Check sheet for the modelled part. Datum: model origin and axes. Units: mm. A direction names the side the tool comes from. Give positions to 0.01 mm unless a question says otherwise; leave off trailing zeros. Write each loop counter-clockwise with the first axis right and the second up, starting at its lowest first coordinate (ties: lowest second). Pieces come first, ordered by that corner, then holes. Notation, with made-up numbers: M 19.5,59 L 31.5,59 A16 ccw 31.5,66 Z; hole C 5,-13 d8. An arc over 180 degrees is marked long. Use CSV: the item, a comma, the result in double quotes. Start each with the question number.
1. Scan lines: line 1 (X direction, y = 7.25, z = 87.5); line 2 (Z direction, x = -2.5, y = 5.5); line 3 (X direction, y = 3.75, z = 87.5). Record each from-to range of solid material in increasing order.
2. Mould release check, pull along Z, two halves, no side actions. Record for faces 1 (the face through (23, 5.2, 49)), 2 (the face through (6, 5, 100)), 3 (the face through (-2.41, 4.93, 85.14)): +Z half, -Z half, draft (parallel to the pull), parting line (faces both ways), or undercut.
3. Cross-section at C-C, the plane z = 76. Enter the section's corners in (x, y).
4. Access from +Z, -Z, +X, -X, +Y, -Y to the whole of each face (thin tool, end or side, straight path). Record for faces 4 (the face through (17.32, 2.56, 98.5)), 5 (the face through (18.75, 3, 49)), 6 (the face through (17.25, 2.56, 1.43)).
5. Cross-section at B-B, the plane y = 7.5. Enter the section's corners in (x, z).
6. Cross-section at D-D, the plane z = 13. Enter the section's corners in (x, y), and give its area (3 significant figures).
7. Cross-section at A-A, the plane z = 87.5. Enter the section's corners in (x, y).
8. Depth check by flat-ended pin: P1, Ø12.5, axis at x = 18, z = 51.5, coming from the -Y side; P2, Ø5, axis at x = -0.25, z = 87.5, coming from the -Y side; P3, Ø3, axis at y = 1, z = 36.5, coming from the +X side. Enter the tip coordinate at first touch or a pass-through.
Autodesk Inventor part; units mm, degrees
ref_plane "YZ Plane" through (0, 0, 0) normal (1, 0, 0) x (0, 1, 0)
ref_plane "XZ Plane" through (0, 0, 0) normal (0, 1, 0) x (-1, 0, 0)
ref_plane "XY Plane" through (0, 0, 0) normal (0, 0, 1) x (1, 0, 0)
sketch "Skizze1" plane through (0, 0, 0) normal (0, 0, 1) x (1, 0, 0)
  line L0 (-10.2503, 0) -> (-10.2503, 10)
  line L1 (-10.2503, 10) -> (29.2497, 10)
  line L2 (29.2497, 10) -> (29.2497, 5.2)
  line L3 (29.2497, 5.2) -> (18.7497, 5.2)
  line L4 (18.7497, 5.2) -> (18.7497, 0)
  line L5 (18.7497, 0) -> (-10.2503, 0)
  point P0 (0, 0)
  dimension "d0" = 39.5
  dimension "d1" = 10
  dimension "d2" = 5.2
  dimension "d5" = 10.5
extrude "Extrusion1" add sketch "Skizze1" along normal blind 100
sketch "Skizze2" plane through (-10.2503, 10, 0) normal (0, 1, 0) x (1, 0, 0)
  line L0 (0, 0) -> (0, -100)
  line L1 (39.5, 0) -> (39.5, -100)
  line L2 (39.5, -100) -> (0, -100)
  point P0 (10.2503, 0)
  point P1 (10, -37.5)
  point P2 (10, -62.5)
  point P3 (10, -87.5)
  point P4 (10, -12.5)
  dimension "d10" = 10
  dimension "d11" = 10
  dimension "d12" = 10
  dimension "d13" = 12.5
  dimension "d14" = 25
  dimension "d15" = 25
  dimension "d16" = 10
  dimension "d17" = 25
hole "Bohrung1" at (-0.2503, 10, 37.5) at (-0.2503, 10, 62.5) at (-0.2503, 10, 87.5) at (-0.2503, 10, 12.5) direction (0, -1, 0) diameter 6.4 end through all
fillet "Rundung1" radius 5 6 edges at (-10.2503, 5, 0) (-10.2503, 5, 100) (29.2497, 7.6, 0) (18.7497, 2.6, 0) (29.2497, 7.6, 100) (18.7497, 2.6, 100)
properties part number "FMR_DXWD80_CPW_Halter_D"
Worked answers:
1,line 1,"x = -10.25 to -3.45, 2.95 to 29.25"
1,line 2,"z = 0 to 10.22, 14.78 to 35.22, 39.78 to 60.22, 64.78 to 85.22, 89.78 to 100"
1,line 3,"x = -10.25 to -3.45, 2.95 to 18.75"
2,face 1,"draft"
2,face 2,"+Z half"
2,face 3,"undercut"
3,outline,"M -10.25,0 L 18.75,0 L 18.75,5.2 L 29.25,5.2 L 29.25,10 L -10.25,10 Z"
4,face 4,"+Z, +X, -Y"
4,face 5,"+Z, -Z, +X, -Y"
4,face 6,"-Z, +X, -Y"
5,outline,"M -10.25,5 A5 ccw -5.25,0 L 24.25,0 A5 ccw 29.25,5 L 29.25,95 A5 ccw 24.25,100 L -5.25,100 A5 ccw -10.25,95 Z; hole C -0.25,12.5 d6.4; hole C -0.25,37.5 d6.4; hole C -0.25,62.5 d6.4; hole C -0.25,87.5 d6.4"
6,outline,"M -10.25,0 L -3.41,0 L -3.41,10 L -10.25,10 Z; M 2.91,0 L 18.75,0 L 18.75,5.2 L 29.25,5.2 L 29.25,10 L 2.91,10 Z"
6,area,"277 mm^2"
7,outline,"M -10.25,0 L -3.45,0 L -3.45,10 L -10.25,10 Z; M 2.95,0 L 18.75,0 L 18.75,5.2 L 29.25,5.2 L 29.25,10 L 2.95,10 Z"
8,P1,"stops at y = 0"
8,P2,"passes through"
8,P3,"stops at x = 18.75"
